from build123d import *

# Parameters (mm, degrees)
F1_DEPTH = 25
F3_DEPTH = 25


with BuildPart() as f1:
    # F0 (on Top) → F1 (new body)
    with BuildSketch(Plane.XY):
        with BuildLine():
            ThreePointArc((-10.4646871668, 3.3897378218), (1.7158731254, 10.8653476437), (11, 0))
            ThreePointArc((11, 0), (10.8653476437, -1.7158731254), (10.4646871668, -3.3897378218))
            ThreePointArc((10.4646871668, -3.3897378218), (11.5303364364, -16.8717211773), (0, -23.9393109523))
            ThreePointArc((0, -23.9393109523), (13.4535838876, -19.8013052461), (22.2561561395, -8.8178298218))
            Line((22.2561561395, -8.8178298218), (22.2834265087, 8.7486862959))
            ThreePointArc((22.2834265087, 8.7486862959), (21.5168684816, 10.4935684883), (20.6139374132, 12.1719428685))
            Line((20.6139374132, 12.1719428685), (20.4327683896, 12.1719428685))
            Line((20.4327683896, 12.1719428685), (20.4327683896, 12.4736756736))
            ThreePointArc((20.4327683896, 12.4736756736), (11.7149350874, 20.8770425293), (0, 23.9393109523))
            ThreePointArc((0, 23.9393109523), (-11.5303364364, 16.8717211773), (-10.4646871668, 3.3897378218))
        make_face()
        with BuildLine():
            ThreePointArc((10.4646871668, -3.3897378218), (-3.3897378218, -10.4646871668), (-10.4646871668, 3.3897378218))
            ThreePointArc((-10.4646871668, 3.3897378218), (-11.5303364364, 16.8717211773), (0, 23.9393109523))
            ThreePointArc((0, 23.9393109523), (-13.4843073091, 19.7803959836), (-22.2834265087, 8.7486862959))
            Line((-22.2834265087, 8.7486862959), (-22.2561561395, -8.8178298218))
            ThreePointArc((-22.2561561395, -8.8178298218), (-13.4535838876, -19.8013052461), (0, -23.9393109523))
            ThreePointArc((0, -23.9393109523), (11.5303364364, -16.8717211773), (10.4646871668, -3.3897378218))
        make_face()
        with BuildLine():
            ThreePointArc((20.6139374132, 12.1719428685), (20.5239074006, 12.3231422082), (20.4327683896, 12.4736756736))
            Line((20.4327683896, 12.4736756736), (20.4327683896, 12.1719428685))
            Line((20.4327683896, 12.1719428685), (20.6139374132, 12.1719428685))
        make_face()
        with BuildLine():
            Line((-22.2561561395, -8.8178298218), (-22.2834265087, 8.7486862959))
            ThreePointArc((-22.2834265087, 8.7486862959), (-22.3171762669, 8.6622313721), (-22.3505905999, 8.5756462558))
            ThreePointArc((-22.3505905999, 8.5756462558), (-22.9180889493, 6.917500111), (-23.3627568452, 5.2222793359))
            ThreePointArc((-23.3627568452, 5.2222793359), (-23.9236754966, -0.865077803), (-22.9245601537, -6.8960242628))
            ThreePointArc((-22.9245601537, -6.8960242628), (-22.876956445, -7.0523381007), (-22.8282869054, -7.2083233721))
            ThreePointArc((-22.8282869054, -7.2083233721), (-22.5565817206, -8.0181812122), (-22.2561561395, -8.8178298218))
        make_face()
        with BuildLine():
            ThreePointArc((-22.3505905999, 8.5756462558), (-22.3171762669, 8.6622313721), (-22.2834265087, 8.7486862959))
            Line((-22.2834265087, 8.7486862959), (-22.2860376354, 10.4306730632))
            Line((-22.2860376354, 10.4306730632), (-26.9655953528, 13.1227395452))
            Line((-26.9655953528, 13.1227395452), (-28.876762415, 14.2222000286))
            Line((-28.876762415, 14.2222000286), (-40.3201948997, 20.8054035902))
            Line((-40.3201948997, 20.8054035902), (-58.3220537256, 10.374730527))
            Line((-58.3220537256, 10.374730527), (-58.2897552873, -10.4306730632))
            Line((-58.2897552873, -10.4306730632), (-40.2555980231, -20.8054035902))
            Line((-40.2555980231, -20.8054035902), (-26.7618837097, -12.9868486414))
            Line((-26.7618837097, -12.9868486414), (-23.1227707365, -10.8782665205))
            Line((-23.1227707365, -10.8782665205), (-22.2537391971, -10.374730527))
            Line((-22.2537391971, -10.374730527), (-22.2561561395, -8.8178298218))
            ThreePointArc((-22.2561561395, -8.8178298218), (-22.5565817206, -8.0181812122), (-22.8282869054, -7.2083233721))
            ThreePointArc((-22.8282869054, -7.2083233721), (-22.876956445, -7.0523381007), (-22.9245601537, -6.8960242628))
            ThreePointArc((-22.9245601537, -6.8960242628), (-23.9236754966, -0.865077803), (-23.3627568452, 5.2222793359))
            ThreePointArc((-23.3627568452, 5.2222793359), (-22.9180889493, 6.917500111), (-22.3505905999, 8.5756462558))
        make_face()
        with BuildLine():
            Line((22.2834265087, 8.7486862959), (22.2561561395, -8.8178298218))
            ThreePointArc((22.2561561395, -8.8178298218), (22.6061950021, -7.8772175544), (22.9165006409, -6.9227600889))
            Line((22.9165006409, -6.9227600889), (22.9165006409, -6.5203195466))
            Line((22.9165006409, -6.5203195466), (23.0342362991, -6.5203195466))
            ThreePointArc((23.0342362991, -6.5203195466), (23.7119627423, -3.291417898), (23.9393109523, 0))
            ThreePointArc((23.9393109523, 0), (23.5915816395, 4.0654501127), (22.5584955519, 8.0127952242))
            Line((22.5584955519, 8.0127952242), (22.2926987152, 8.0127952242))
            Line((22.2926987152, 8.0127952242), (22.2926987152, 8.7250325423))
            ThreePointArc((22.2926987152, 8.7250325423), (22.2880657498, 8.7368606491), (22.2834265087, 8.7486862959))
        make_face()
        with BuildLine():
            ThreePointArc((22.9165006409, -6.9227600889), (22.6061950021, -7.8772175544), (22.2561561395, -8.8178298218))
            Line((22.2561561395, -8.8178298218), (22.2537391971, -10.374730527))
            Line((22.2537391971, -10.374730527), (23.1227707365, -10.8782665205))
            Line((23.1227707365, -10.8782665205), (26.7618837097, -12.9868486414))
            Line((26.7618837097, -12.9868486414), (40.2555980231, -20.8054035902))
            Line((40.2555980231, -20.8054035902), (58.2897552873, -10.4306730632))
            Line((58.2897552873, -10.4306730632), (58.3220537256, 10.374730527))
            Line((58.3220537256, 10.374730527), (40.3201948997, 20.8054035902))
            Line((40.3201948997, 20.8054035902), (28.876762415, 14.2222000286))
            Line((28.876762415, 14.2222000286), (28.9680806238, 14.2222000286))
            Line((28.9680806238, 14.2222000286), (28.9680806238, 12.1719428685))
            Line((28.9680806238, 12.1719428685), (40.3201948997, 18.6999721072))
            Line((40.3201948997, 18.6999721072), (56.4986965755, 9.3220147855))
            Line((56.4986965755, 9.3220147855), (56.4663981371, -9.3779573217))
            Line((56.4663981371, -9.3779573217), (40.2555980231, -18.6999721072))
            Line((40.2555980231, -18.6999721072), (24.0770963473, -9.3220147855))
            Line((24.0770963473, -9.3220147855), (24.0812403203, -6.9227600889))
            Line((24.0812403203, -6.9227600889), (22.9165006409, -6.9227600889))
        make_face()
        with BuildLine():
            Line((22.2860376354, 10.4306730632), (22.2834265087, 8.7486862959))
            ThreePointArc((22.2834265087, 8.7486862959), (22.2880657498, 8.7368606491), (22.2926987152, 8.7250325423))
            Line((22.2926987152, 8.7250325423), (24.1070368889, 8.7250325423))
            Line((24.1070368889, 8.7250325423), (24.1070368889, 8.0127952242))
            Line((24.1070368889, 8.0127952242), (24.1093947856, 9.3779573217))
            Line((24.1093947856, 9.3779573217), (28.9680806238, 12.1719428685))
            Line((28.9680806238, 12.1719428685), (28.9680806238, 14.2222000286))
            Line((28.9680806238, 14.2222000286), (28.876762415, 14.2222000286))
            Line((28.876762415, 14.2222000286), (26.9655953528, 13.1227395452))
            Line((26.9655953528, 13.1227395452), (22.2860376354, 10.4306730632))
        make_face()
    extrude(amount=F1_DEPTH)

    # F2 (on face) → F3 (cut)
    with BuildSketch(Plane.XY.offset(25)):
        Polygon((-56.1096642619, -8.8687674562), (-40.7759704459, -17.6899693007), (-25.4697386486, -8.8212018445), (-25.4972006673, 8.8687674562), (-40.8308944833, 17.6899693007), (-56.1371262806, 8.8212018445), align=None)
    extrude(amount=-F3_DEPTH, mode=Mode.SUBTRACT)


solid = f1.part
Verification items for the finished model (mm, model axes). A direction names the side the tool comes from. Coordinates: 2 decimals unless noted, no trailing zeros. Order: outer loops, then holes, each group sorted by start corner. A loop starts at its lowest first (then second) coordinate and runs counter-clockwise, first axis right, second up. Notation, with made-up numbers: (-23, 20.25) -> (-4, 20.25) arc R31 cw to (-4, 55.25) -> close; hole circle Ø4 at (-1.75, 77.25). An arc over 180 degrees is marked (long way). Put each result on its own line as item: value. Start each with the question number.
1. Access from +Z, -Z, +X, -X, +Y, -Y to the whole of each face (thin tool, end or side, straight path). Record for faces 1 (the flat face through (-33.06, 13.22, 12.68)), 2 (the flat face through (-49.2, 15.66, 12.32)).
2. Cross-section at A-A, the plane y = 5.5. Record the boundary of the cut face in (x, z), then the cut area to 3 significant figures.
3. Go/stop test with flat-tipped pins: pin 1 Ø3 at (y, z) = (4.5, 19.5) entering from -X; pin 2 Ø12 at (y, z) = (-19, 14) entering from -X; pin 3 Ø0.6 at (x, z) = (23.5, 7.5) entering from +Y. Record where each tip stops, or that it passes through.
4. Material ranges on L1, parallel to X at y = -6, z = 1.5; L2, parallel to X at y = -11.5, z = 21; L3, parallel to X at y = 10, z = 13.5, recorded low to high. Write a range as [from, to].
5. Cross-section at B-B, the plane x = -35. Record the boundary of the cut face in (y, z), then the cut area to 3 significant figures.
6. Cross-section at C-C, the plane z = 23.75. Count the separate pieces of the cut face and the enclosed holes in it, then the cut area to 3 significant figures.
7. Mould release check, pull along Y, two halves, no side actions. Record for faces 3 (the flat face through (-49.399, -15.545, 12.325)), 4 (the flat face through (32.28, -14.077, 12.325)), 5 (the flat face through (-9, -7, 25)): released by +Y, released by -Y, zero draft, split by the parting line, or undercut.
Computed:
1. face 1: +Z, -Z
1. face 2: +Z, -Z, -X, +Y
2. outline: (-58.31, 0) -> (-56.13, 0) -> (-56.13, 25) -> (-58.31, 25) -> close; (-25.49, 0) -> (-9.53, 0) -> (-9.53, 25) -> (-25.49, 25) -> close; (9.53, 0) -> (23.3, 0) -> (23.3, 25) -> (9.53, 25) -> close; (56.49, 0) -> (58.31, 0) -> (58.31, 25) -> (56.49, 25) -> close
2. area: 844 mm2
3. pin 1: x = -58.32
3. pin 2: x = -53.82
3. pin 3: y = 11.3
4. L1: [-58.3, -56.11], [-25.47, -9.22], [9.22, 23.18], [56.47, 58.3]
4. L2: [-56.43, -51.54], [-30.09, -24.2], [-21, 21], [24.2, 27.83], [52.78, 56.43]
4. L3: [-58.32, -54.1], [-27.46, -22.29], [-21.75, -4.58], [4.58, 21.75], [22.29, 25.19], [55.33, 58.32]
5. outline: (-17.76, 0) -> (-14.34, 0) -> (-14.34, 25) -> (-17.76, 25) -> close; (14.34, 0) -> (17.74, 0) -> (17.74, 25) -> (14.34, 25) -> close
5. area: 171 mm2
6. separate pieces: 1
6. enclosed holes: 3
6. area: 1,900 mm2
7. face 3: released by -Y
7. face 4: undercut
7. face 5: zero draft
